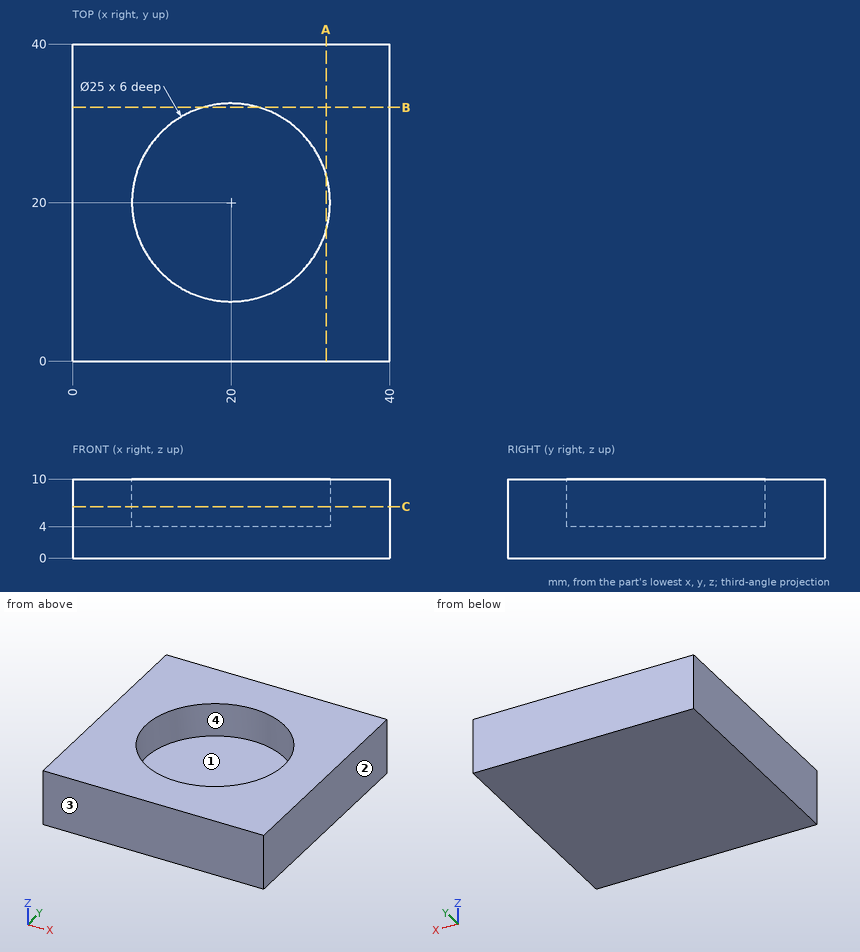
Answer from the drawing. Dimensions are ordinates in mm from the lowest x, y and z of the part. Coordinates: 2 decimals unless noted, no trailing zeros. Order: outer loops, then holes, each group sorted by start corner. A loop starts at its lowest first (then second) coordinate and runs counter-clockwise, first axis right, second up. Notation, with made-up numbers: (-30.75, 5) - (-25.75, 5) arc R10 ccw to (-25.75, 16) - close; hole circle Ø8 at (43.5, 49). An arc over 180 degrees is marked (long way). Put each result on its own line as item: value. Start each with the question number.
1) Find section A-A (x = 32). Give the vertices of the cut face in (y, z).
2) Find the intervals of material crossed by line 1 (Y direction, x = 20, z = 6.85); line 2 (Z direction, x = 27, y = 15); line 3 (Y direction, x = 30, z = 9.75), in increasing order. Write a range as from..to.
3) Find section C-C (z = 6.5). Give the vertices of the cut face in (x, y), plus the area to 3 significant figures.
4) For a pull along X with two mould halves and no side action, classify the marked faces 1, 2, 3 and 4 as released by +X, released by -X, zero draft, split by the parting line, or undercut.
5) Flat-ended cylindrical pins translate along their axes: pin 1 (6 mm diameter, centred on x = 29.5, y = 23, fed in from +Z); pin 2 (7.5 mm diameter, centred on x = 23, y = 21, fed in from +Z). Find the tip coordinate at first contact, or state that the pin passes through.
Results list:
1. outline: (0, 0) - (40, 0) - (40, 10) - (23.5, 10) - (23.5, 4) - (16.5, 4) - (16.5, 10) - (0, 10) - close
2. line 1: y = 0..7.5, 32.5..40
2. line 2: z = 0..4
2. line 3: y = 0..12.5, 27.5..40
3. outline: (0, 0) - (40, 0) - (40, 40) - (0, 40) - close; hole circle Ø25 at (20, 20)
3. area: 1,110 mm^2
4. face 1: undercut
4. face 2: released by +X
4. face 3: zero draft
4. face 4: undercut
5. pin 1: stops at z = 10
5. pin 2: stops at z = 4
